Part model, mm, in its own coordinate system. A direction names the side the tool comes from. Round coordinates to 2 decimals unless told otherwise and drop trailing zeros. Write each loop counter-clockwise with the first axis right and the second up, starting at its lowest first coordinate (ties: lowest second). Pieces come first, ordered by that corner, then holes. Notation, with made-up numbers: (50.25, 2) -> (78.25, 2) arc R17 cw to (78.25, 11) -> close; hole circle Ø8 at (68.25, 61). An arc over 180 degrees is marked (long way). Return JSON: item names as keys, results as strings. Group by question number.
```python
from build123d import *

# Parameters (mm, degrees)
SKETCH1_R           = 11.75
BOSS_EXTRUDE1_DEPTH = 0.6
SKETCH2_R           = 11.75
SKETCH2_R_2         = 9.75
BOSS_EXTRUDE2_DEPTH = 1.6
BOSS_EXTRUDE3_DEPTH = 1.6
FILLET1_R           = 1


with BuildPart() as part:
    # Sketch1 → Boss-Extrude1 (new body)
    with BuildSketch(Plane.XY):
        Circle(SKETCH1_R)
    extrude(amount=BOSS_EXTRUDE1_DEPTH)

    # Sketch2 → Boss-Extrude2 (add)
    with BuildSketch(Plane.XY.offset(0.6)):
        Circle(SKETCH2_R)
        Circle(SKETCH2_R_2, mode=Mode.SUBTRACT)
    extrude(amount=BOSS_EXTRUDE2_DEPTH)

    # Sketch3 → Boss-Extrude3 (add)
    with BuildSketch(Plane.XY.offset(0.6)):
        with BuildLine():
            Line((-6.916956338, -0.911963991), (-5.361151216, -0.911963991))
            add(Edge.make_bspline(
                [(-5.361151216, -0.911963991), (-5.239855358, -0.911135682), (-5.005389093, -0.909534551), (-4.665741882, -0.890804083), (-4.349677023, -0.863299234), (-4.057909505, -0.821204302), (-3.789388655, -0.772346551), (-3.546096572, -0.706915643), (-3.326053246, -0.631828045), (-3.126949332, -0.544340632), (-2.945683277, -0.44173815), (-2.7747857, -0.326468517), (-2.612283679, -0.196802417), (-2.45727666, -0.052438003), (-2.309386888, 0.10566485), (-2.172085953, 0.280689674), (-2.040972084, 0.468103096), (-1.918172617, 0.668555578), (-1.808865755, 0.881651378), (-1.711570392, 1.104036522), (-1.630505782, 1.335855545), (-1.564500099, 1.576788364), (-1.511922924, 1.826137054), (-1.475126432, 2.084376718), (-1.452380824, 2.351276025), (-1.4500733, 2.532166496), (-1.448900782, 2.624082016)],
                knots=[0, 0, 0, 0, 0.000363844, 0.000703314, 0.001020209, 0.001315264, 0.001587422, 0.001838456, 0.002070302, 0.002284378, 0.002489835, 0.002694315, 0.002902211, 0.00311283, 0.003329292, 0.003550963, 0.003779572, 0.004015201, 0.004255569, 0.004497496, 0.004742868, 0.004991603, 0.005246465, 0.005506831, 0.005773705, 0.006049398, 0.006049398, 0.006049398, 0.006049398], degree=3))
            add(Edge.make_bspline(
                [(-1.448900782, 2.624082016), (-1.451970756, 2.753780967), (-1.458014179, 3.009100945), (-1.508926104, 3.383777758), (-1.591254497, 3.742951732), (-1.707062559, 4.083771806), (-1.850470901, 4.403352066), (-2.022220096, 4.695290765), (-2.217376545, 4.960182986), (-2.437672033, 5.19363362), (-2.675821661, 5.395516124), (-2.924276522, 5.566399637), (-3.182814338, 5.703564799), (-3.41110213, 5.789220823), (-3.609613669, 5.843055986), (-3.783646836, 5.874330612), (-3.981711628, 5.903336547), (-4.204554541, 5.928267914), (-4.452836402, 5.945340974), (-4.725788377, 5.957131127), (-5.023476578, 5.965891962), (-5.23023053, 5.966754323), (-5.337724567, 5.967202676)],
                knots=[0, 0, 0, 0, 0.000388958, 0.000765687, 0.001132051, 0.001492876, 0.0018438, 0.002181059, 0.002507107, 0.002828814, 0.003141656, 0.003442084, 0.0037318, 0.004017439, 0.00417154, 0.004348294, 0.004547467, 0.004772083, 0.005020776, 0.005293909, 0.005591681, 0.005914153, 0.005914153, 0.005914153, 0.005914153], degree=3))
            Line((-5.337724567, 5.967202676), (-6.916956338, 5.967202676))
            Line((-6.916956338, 5.967202676), (-6.916956338, -0.911963991))
        make_face()
        with BuildLine():
            Line((-5.682234116, 0.322758231), (-5.682234116, 4.732480453))
            Line((-5.682234116, 4.732480453), (-5.037312241, 4.732480453))
            add(Edge.make_bspline(
                [(-5.037312241, 4.732480453), (-4.960589746, 4.732108932), (-4.813049194, 4.73139448), (-4.599773783, 4.721578003), (-4.402949586, 4.705637209), (-4.222318791, 4.682058374), (-4.05746614, 4.653687), (-3.90899297, 4.61859535), (-3.776606644, 4.575921232), (-3.659215448, 4.525629351), (-3.552039877, 4.468210013), (-3.452750381, 4.401161931), (-3.356923903, 4.32665025), (-3.266331588, 4.24255096), (-3.180635874, 4.149959395), (-3.100343516, 4.048403256), (-3.024378224, 3.938192199), (-2.954709427, 3.818739134), (-2.890985622, 3.691323934), (-2.834687293, 3.557108901), (-2.787161197, 3.415362356), (-2.751069756, 3.266147042), (-2.720324605, 3.110388904), (-2.698124248, 2.947086468), (-2.686029416, 2.77677325), (-2.684432963, 2.66084794), (-2.683623005, 2.602033405)],
                knots=[0, 0, 0, 0, 0.000230149, 0.000442586, 0.000640338, 0.000822375, 0.000988895, 0.001141975, 0.001279683, 0.00140562, 0.001524619, 0.001643866, 0.001764607, 0.001888454, 0.002014249, 0.002142732, 0.002276515, 0.002415486, 0.002557229, 0.00270362, 0.002851783, 0.003005191, 0.003163833, 0.00332793, 0.003499256, 0.003675693, 0.003675693, 0.003675693, 0.003675693], degree=3))
            add(Edge.make_bspline(
                [(-2.683623005, 2.602033405), (-2.685262463, 2.511908699), (-2.688459279, 2.336172506), (-2.719481404, 2.080243078), (-2.769467097, 1.839548826), (-2.842282437, 1.614708069), (-2.931826264, 1.404291395), (-3.045683112, 1.211010286), (-3.176936165, 1.031696657), (-3.280787507, 0.926524812), (-3.332678994, 0.873973509)],
                knots=[0, 0, 0, 0, 0.000270268, 0.000527001, 0.000772141, 0.001006602, 0.001234957, 0.001456654, 0.001678245, 0.001899543, 0.001899543, 0.001899543, 0.001899543], degree=3))
            add(Edge.make_bspline(
                [(-3.332678994, 0.873973509), (-3.383844652, 0.829191175), (-3.488344714, 0.737728328), (-3.671812484, 0.628132448), (-3.873984463, 0.531841725), (-4.099485742, 0.455493921), (-4.346136951, 0.395114822), (-4.615407148, 0.353472834), (-4.905854335, 0.326714134), (-5.107069378, 0.324105116), (-5.210945053, 0.322758231)],
                knots=[0, 0, 0, 0, 0.000203614, 0.000415859, 0.00063839, 0.000874594, 0.001128605, 0.001399336, 0.001691279, 0.002002825, 0.002002825, 0.002002825, 0.002002825], degree=3))
            Line((-5.210945053, 0.322758231), (-5.682234116, 0.322758231))
        make_face(mode=Mode.SUBTRACT)
        Polygon((6.248715571, 1.676089617), (4.96714005, 1.676089617), (3.397554546, -3.122239376), (1.816944737, 1.676089617), (0.54777156, 1.676089617), (-0.615292676, -5.20307705), (0.634587966, -5.20307705), (1.369082324, -0.858122623), (2.79948597, -5.20307705), (4.003891352, -5.20307705), (5.426026769, -0.858122623), (6.159143088, -5.20307705), (7.410401769, -5.20307705), align=None)
    extrude(amount=BOSS_EXTRUDE3_DEPTH)

    # Fillet1
    fillet1_edges = [part.edges().sort_by_distance(p)[0] for p in [
        (-11.75, 0, 2.2),
    ]]
    fillet(fillet1_edges, radius=FILLET1_R)


solid = part.part
```
Item 1: Cut at A-A (x = 0). Write the cut outline in (y, z), then the cut area to 3 significant figures.
Item 2: Flat gauge pins, fed straight in: P1, Ø0.8, axis at y = 2, z = 1.5, coming from the +X side; P2, Ø0.7, axis at x = -5, z = 1.5, coming from the -Y side; P3, Ø1, axis at x = 6, z = 1.5, coming from the +Y side. Where does each tip first touch, or does it go through?
Item 3: Cut at B-B (z = 1.55). State how many separate pieces and enclosed holes the cut face has, then the cut area to 3 significant figures.
Item 4: Which spindle directions (+Z, -Z, +X, -X, +Y, -Y) get a long thin tool onto all of the face, cutting with end or side? Do faces 1 (the face through (0, -5.203, 1)), 2 (the face through (-6, 3, 2.2)). Say none if no direction does.
Item 5: Two-plate mould, pull along X, no slides. Class faces 3 (the face through (2, -10, 2.2)), 4 (the face through (-6, -0.912, 1)): released by +X, released by -X, zero draft, split by the parting line, or undercut.
Item 6: Wall check: L1, parallel to Y at x = -5.5, z = 0.65; L2, parallel to X at y = 1.5, z = 1; L3, parallel to Z at x = -1.75, y = -5. Give the ranges that are in metal, low to high.
Checks:
{
 "1": {"outline": "(-11.75, 0) -> (11.75, 0) -> (11.75, 1.2) arc R1 ccw to (10.75, 2.2) -> (9.75, 2.2) -> (9.75, 0.6) -> (-1.56, 0.6) -> (-1.56, 2.2) -> (-5.2, 2.2) -> (-5.2, 0.6) -> (-9.75, 0.6) -> (-9.75, 2.2) -> (-10.75, 2.2) arc R1 ccw to (-11.75, 1.2) -> close", "area": "25.9 mm2"},
 "2": {"P1": "stops at x = 11.63", "P2": "stops at y = -10.76", "P3": "stops at y = 10.36"},
 "3": {"separate pieces": "3", "enclosed holes": "2", "area": "182 mm2"},
 "4": {"face 1": "+Z", "face 2": "+Z, +X, -X, +Y, -Y"},
 "5": {"face 3": "zero draft", "face 4": "undercut"},
 "6": {"L1": "y = -10.38 to -8.05, -0.91 to 0.32, 4.73 to 5.97, 8.05 to 10.38", "L2": "x = -11.65 to -9.63, -6.92 to -5.68, -2.89 to -1.59, 0.52 to 1.87, 4.91 to 6.28, 9.63 to 11.65", "L3": "z = 0 to 0.6"}
}
